from build123d import *

# Parameters (mm, degrees)
FILLET1_R = 1


with BuildPart() as part:
    # Sketch1 → Revolve3 (revolve)
    with BuildSketch(Plane.XY.offset(84.279), mode=Mode.PRIVATE) as revolve3_sk:
        Polygon((-115.072, 105.221), (-109.230578644, 105.221), (-102.830578644, 111.621), (-88.572, 111.621), (-88.572, 107.621), (-96.272, 107.621), (-101.072, 102.821), (-115.072, 102.821), align=None)
    revolve(revolve3_sk.sketch.rotate(Axis((-96.072, 102.821, 84.279), (1, 0, 0)), 90), axis=Axis((-96.072, 102.821, 84.279), (1, 0, 0)))

    # Fillet1
    fillet1_edges = [part.edges().sort_by_distance(p)[0] for p in [
        (-109.230578644, 102.821, 81.879),
        (-102.830578644, 102.821, 75.479),
        (-88.572, 102.821, 75.479),
    ]]
    fillet(fillet1_edges, radius=FILLET1_R)


solid = part.part
Model file for the job. Use its own axes, mm. A direction names the side the tool comes from. Coordinates: 2 decimals unless noted, no trailing zeros. Write each loop counter-clockwise with the first axis right and the second up, starting at its lowest first coordinate (ties: lowest second). Pieces come first, ordered by that corner, then holes. Notation, with made-up numbers: (70, 14) -> (80, 14) arc R19 ccw to (80, 30) -> close; hole circle Ø8 at (2.25, 73.5). An arc over 180 degrees is marked (long way). One line per item, written item: value. Start each with the question number.
1) Which spindle directions (+Z, -Z, +X, -X, +Y, -Y) get a long thin tool onto all of the face, cutting with end or side? Do faces 1 (the face through (-92.476, 104.659, 88.713)), 2 (the face through (-108.574, 101.903, 87.194)). Say none if no direction does.
2) Slice it at C-C on x = -97. Write the cut outline in (y, z), then the cut area to 3 significant figures.
3) Slice it at B-B on x = -112.5. Write the cut outline in (y, z), then the cut area to 3 significant figures.
4) Probe probe 1 along Z at (x, y) = (-94.25, 99.75); probe 2 along Y at (x, z) = (-94, 83); probe 3 along Z at (x, y) = (-90.25, 106). List the from-to ranges inside material, lowest first.
5) Pull direction Y, two halves, no side cores. Call faces 3 (the face through (-112.32, 102.1, 86.57)), 4 (the face through (-99.772, 101.725, 84.978)), 5 (the face through (-115.072, 103, 84)): +Y half, -Y half, draft (parallel to the pull), parting line (faces both ways), or undercut.
6) Slice it at D-D on x = -106.25. Write the cut outline in (y, z).
7) Slice it at A-A on x = -92.5. Write the cut outline in (y, z).
8) Flat gauge pins, fed straight in: pin 1 Ø1 at (y, z) = (104.5, 81) entering from -X; pin 2 Ø1 at (x, y) = (-111, 102) entering from -Z; pin 3 Ø10 at (y, z) = (101, 87.5) entering from -X; pin 4 Ø1.5 at (x, z) = (-108.5, 85) entering from +Y (3 decimals). Where does each tip first touch, or does it go through?
Answers follow:
1. face 1: +X
1. face 2: -X
2. outline: circle Ø17.6 at (102.82, 84.28); hole circle Ø8.14 at (102.82, 84.28)
2. area: 191 mm2
3. outline: circle Ø4.8 at (102.82, 84.28)
3. area: 18.1 mm2
4. probe 1: 76.03 to 80.59, 87.97 to 92.53
4. probe 2: 94.11 to 98.19, 107.45 to 111.53
4. probe 3: 76.07 to 80.68, 87.88 to 92.48
5. face 3: parting line
5. face 4: undercut
5. face 5: draft
6. outline: circle Ø10.76 at (102.82, 84.28)
7. outline: circle Ø17.6 at (102.82, 84.28); hole circle Ø9.6 at (102.82, 84.28)
8. pin 1: x = -108.45
8. pin 2: z = 81.9
8. pin 3: x = -115.07
8. pin 4: y = 106.645
